Can you work these out from the model? Positions are in its coordinate system, mm. Round coordinates to 2 decimals unless told otherwise and drop trailing zeros. Loops run counter-clockwise (first coordinate to the right, second up) from the corner with the lowest first, then second, coordinate; pieces in that order, holes last. Notation, with made-up numbers: (19, 86) -> (67, 86) arc R18 ccw to (67, 106) -> close; hole circle Ø9 at (-9.75, 44.25). An arc over 180 degrees is marked (long way). Answer as a JSON object with one key per item and string values.
```python
from build123d import *

# Parameters (mm, degrees)
FILLET1_R       = 0.1
HEX_START       = -1.1
HEX_2_DEPTH     = 1.1
THDSCHPAT_COUNT = 35
THDSCHPAT_PITCH = 0.489714286


with BuildPart() as part:
    # BodySke → BaseBody (revolve)
    with BuildSketch(Plane.XY, mode=Mode.PRIVATE) as basebody_sk:
        Polygon((0, 0), (0, 2.675), (0.685, 2.675), (1.86, 1.5), (19.7195, 1.5), (20, 1.2195), (20, 0), align=None)
    revolve(basebody_sk.sketch.rotate(Axis((0, 0, 0), (1, 0, 0)), 90), axis=Axis((0, 0, 0), (1, 0, 0)))

    # Fillet1
    fillet1_edges = [part.edges().sort_by_distance(p)[0] for p in [
        (1.86, 0, -1.5),
    ]]
    fillet(fillet1_edges, radius=FILLET1_R)

    # Hex 2: read off the stored shape, not the designer's step
    # Hex 2 outline → Hex 2 (cut)
    with BuildSketch(Plane.ZY.offset(HEX_START)):
        Polygon((-1, -0.577350269), (0, -1.154700538), (1, -0.577350269), (1, 0.577350269), (0, 1.154700538), (-1, 0.577350269), align=None)
    extrude(amount=HEX_2_DEPTH, mode=Mode.SUBTRACT)

    # Hex 2 2 outline → Hex 2 2 (revolve, cut)
    with BuildSketch(Plane.YX):
        Polygon((1, 1.1), (0, 1.677350269), (0, 1.1), align=None)
    revolve(axis=Axis((0, 0, 0), (1, 0, 0)), mode=Mode.SUBTRACT)

    # ThdSchSke → ThreadSchematic (revolve, cut)
    with BuildSketch(Plane.XY, mode=Mode.PRIVATE) as threadschematic_sk:
        Polygon((2.860001, -1.2195), (2.663592786, -1.5), (2.663592786, -1.875), (3.056409214, -1.875), (3.056409214, -1.5), align=None)
    threadschematic = revolve(threadschematic_sk.sketch.rotate(Axis((-3.175, 0, 0), (1, 0, 0)), 270), axis=Axis((-3.175, 0, 0), (1, 0, 0)), mode=Mode.SUBTRACT)

    # ThdSchPat: ThreadSchematic ×35
    with Locations(*[(i * THDSCHPAT_PITCH, 0, 0) for i in range(1, THDSCHPAT_COUNT)]):
        add(threadschematic, mode=Mode.SUBTRACT)


solid = part.part
```
Q1. I want a section at A-A, the plane x = 2.25. Write out the boundary of the cut face in (y, z).
Determined:
{"outline": "circle Ø3 at (0, 0)"}
Q2. If I drill on L1, parallel to Y at x = 9, z = 1.3; L2, parallel to Y at x = 12.5, z = -1.15; L3, parallel to X at y = -1.55, z = -0.2, over which ranges is the centre line in solid material (lowest first)? Write a range as [from, to].
Determined:
{"L1": "[-0.75, 0.75]", "L2": "[-0.87, 0.87]", "L3": "[0, 1.8]"}
Q3. I'm going to push a flat-ended pin straight in: pin 1 (1.5 mm diameter, centred on x = 10.5, z = 0, fed in from -Y). Where does the tip first touch, or does it pass through?
Determined:
{"pin 1": "y = -1.5"}
